Source: three-view drawing plus pictorial views. Frame: mm from the lowest corner of the part. Round coordinates to 2 decimals unless told otherwise and drop trailing zeros. Write each loop counter-clockwise with the first axis right and the second up, starting at its lowest first coordinate (ties: lowest second). Pieces come first, ordered by that corner, then holes. Notation, with made-up numbers: M -33.5,-20 L -9.5,-20 A19 cw -9.5,-15 Z; hole C 5,-38 d4. An arc over 180 degrees is marked long. Answer in a Markdown table with one row per item.
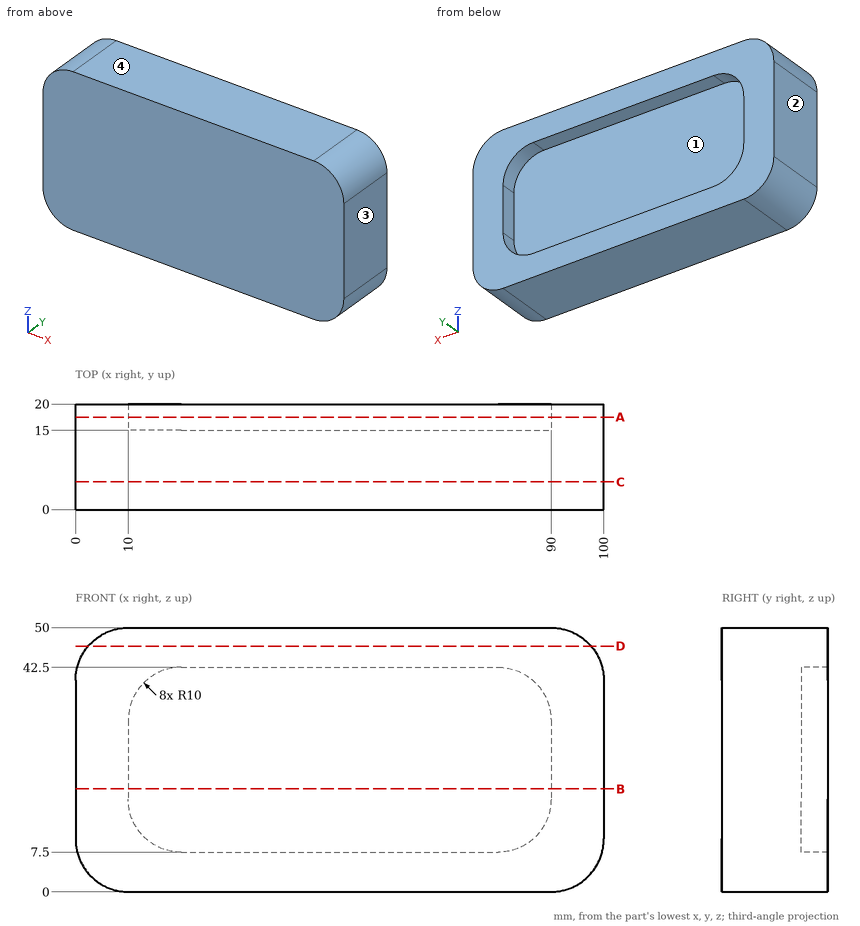
Q1. Pull-direction query (X, two-part tool) for the marked faces 1, 2, 3 and 4; classes: pulls with the +X half, pulls with the -X half, needs draft (parallel to the pull), parting line crosses it, or undercut.
Solutions:
| item | result |
|---|---|
| face 1 | undercut |
| face 2 | pulls with the -X half |
| face 3 | pulls with the +X half |
| face 4 | needs draft |
Q2. Section D-D (z = 46.5). Return loops of the section in (x, y).
Solutions:
| item | result |
|---|---|
| outline | M 2.4,0 L 97.6,0 L 97.6,20 L 2.4,20 Z |
Q3. Material intervals for probe 1 along Z at (x, y) = (19.5, 17); probe 2 along X at (y, z) = (18.5, 29); probe 3 along Y at (x, z) = (70.5, 39), sorted ascending.
Solutions:
| item | result |
|---|---|
| probe 1 | z = 0 to 7.51, 42.49 to 50 |
| probe 2 | x = 0 to 10, 90 to 100 |
| probe 3 | y = 0 to 15 |
Q4. Contact query for flat-ended pins moving along their axis: pin 1 Ø8 at (x, z) = (35, 15) entering from -Y; pin 2 Ø6 at (x, z) = (27, 30) entering from +Y. Output: stop coordinate, or through.
Solutions:
| item | result |
|---|---|
| pin 1 | stops at y = 0 |
| pin 2 | stops at y = 15 |
Q5. Section C-C (y = 5.25). Return loops of the section in (x, z).
Solutions:
| item | result |
|---|---|
| outline | M 0,10 A10 ccw 10,0 L 90,0 A10 ccw 100,10 L 100,40 A10 ccw 90,50 L 10,50 A10 ccw 0,40 Z |
Q6. Section B-B (z = 19.5). Return loops of the section in (x, y), and give its area (3 significant figures).
Solutions:
| item | result |
|---|---|
| outline | M 0,0 L 100,0 L 100,20 L 90,20 L 90,15 L 10,15 L 10,20 L 0,20 Z |
| area | 1,600 mm2 |
Q7. Section A-A (y = 17.5). Return loops of the section in (x, z).
Solutions:
| item | result |
|---|---|
| outline | M 0,10 A10 ccw 10,0 L 90,0 A10 ccw 100,10 L 100,40 A10 ccw 90,50 L 10,50 A10 ccw 0,40 Z; hole M 10,17.5 A10 ccw 20,7.5 L 80,7.5 A10 ccw 90,17.5 L 90,32.5 A10 ccw 80,42.5 L 20,42.5 A10 ccw 10,32.5 Z |
